Work out the finished part from the listing and answer in its coordinate system (mm). Face numbers are marked on the shaded views. A direction names the side the tool comes from. Coordinates: 2 decimals unless noted, no trailing zeros. Write each loop counter-clockwise with the first axis right and the second up, starting at its lowest first coordinate (ties: lowest second). Pieces come first, ordered by that corner, then holes. Notation, with made-up numbers: M 56.5,87.5 L 82.5,87.5 A23 cw 82.5,99.5 Z; hole C 43,39.25 d11. An arc over 180 degrees is marked long. Use CSV: the item, a comma, the result in double quotes.
from build123d import *

# Parameters (mm, degrees)
SKETCH1_W                    = 250
SKETCH1_H                    = 153
BASE_FLANGE1_DEPTH           = 2.06
EDGE_FLANGE1_STRIP_W         = 10.272
EDGE_FLANGE1_STRIP_H         = 2.06
EDGE_FLANGE1_STRIP_CUT_DEPTH = 250
EDGE_FLANGE1_DEPTH           = 250
EDGE_FLANGE2_DEPTH           = 50
CHAMFER1_SIZE                = 10
SKETCH13_R                   = 2
CUT_EXTRUDE2_DEPTH           = 8.4
SKETCH14_R                   = 2.25
CUT_EXTRUDE3_DEPTH           = 8.4
SKETCH20_W                   = 73
SKETCH20_H                   = 64
CUT_EXTRUDE9_DEPTH           = 10
FILLET1_R                    = 10
CHAMFER3_SIZE                = 15
CHAMFER4_SIZE                = 15
SKETCH21_R                   = 1.5
CUT_EXTRUDE10_DEPTH          = 10
FILLET2_R                    = 5
CUT_EXTRUDE11_DEPTH          = 10
CHAMFER5_SIZE                = 5


# Sheet-metal steps are written as plain solids
with BuildPart() as part:
    # Sketch1 → Base-Flange1 (new body)
    with BuildSketch(Plane.XY):
        with Locations((125, 76.5)):
            Rectangle(SKETCH1_W, SKETCH1_H)
    extrude(amount=-BASE_FLANGE1_DEPTH)

    # Edge-Flange1 strip (across the edge) → Edge-Flange1 strip cut (cut)
    with BuildSketch(Plane.YZ):
        with Locations((-2.06, -1.03)):
            Rectangle(EDGE_FLANGE1_STRIP_W, EDGE_FLANGE1_STRIP_H)
    extrude(amount=EDGE_FLANGE1_STRIP_CUT_DEPTH, mode=Mode.SUBTRACT)

    # Edge-Flange1 section (across the edge) → Edge-Flange1 (add)
    with BuildSketch(Plane.YZ):
        with BuildLine():
            Line((0, 1.016), (0, 15))
            Line((0, 15), (2.06, 15))
            Line((2.06, 15), (2.06, 1.016))
            ThreePointArc((2.06, 1.016), (2.35757951, 0.29757951), (3.076, 0))
            Line((3.076, 0), (3.076, -2.06))
            ThreePointArc((3.076, -2.06), (0.900939541, -1.159060459), (0, 1.016))
        make_face()
    extrude(amount=EDGE_FLANGE1_DEPTH)

    # Edge-Flange2 section (across the edge) → Edge-Flange2 (add)
    with BuildSketch(Plane(origin=(270, 87, 0), x_dir=(-1, 0, 0), z_dir=(0, 1, 0))):
        with BuildLine():
            Line((0, 1.016), (0, 15))
            Line((0, 15), (2.06, 15))
            Line((2.06, 15), (2.06, 1.016))
            ThreePointArc((2.06, 1.016), (2.35757951, 0.29757951), (3.076, 0))
            Line((3.076, 0), (20, 0))
            Line((20, 0), (20, -2.06))
            Line((20, -2.06), (3.076, -2.06))
            ThreePointArc((3.076, -2.06), (0.900939541, -1.159060459), (0, 1.016))
        make_face()
    extrude(amount=EDGE_FLANGE2_DEPTH)

    # Chamfer1
    chamfer1_edges = [part.edges().sort_by_distance(p)[0] for p in [
        (0, 1.03, 15),
        (250, 1.03, 15),
        (250, 87, -1.03),
        (250, 153, -1.03),
    ]]
    chamfer(chamfer1_edges, length=CHAMFER1_SIZE)

    # Sketch13 → Cut-Extrude2 (cut)
    with BuildSketch(Plane(origin=(0, 2.06, 0), x_dir=(1, 0, 0), z_dir=(0, 1, 0))):
        with Locations(Location((125, -8.008, 0), (0, 0, 270))):
            Circle(SKETCH13_R)
        with Locations(Location((235, -8.008, 0), (0, 0, 270))):
            Circle(SKETCH13_R)
        with Locations(Location((15, -8.008, 0), (0, 0, 270))):
            Circle(SKETCH13_R)
    extrude(amount=-CUT_EXTRUDE2_DEPTH, mode=Mode.SUBTRACT)

    # Sketch14 → Cut-Extrude3 (cut)
    with BuildSketch(Plane.ZY.offset(-267.94)):
        with Locations((8.008, 127)):
            Circle(SKETCH14_R)
        with Locations((8.008, 97)):
            Circle(SKETCH14_R)
    extrude(amount=-CUT_EXTRUDE3_DEPTH, mode=Mode.SUBTRACT)

    # Sketch20 → Cut-Extrude9 (cut)
    with BuildSketch(Plane.XY):
        with Locations((36.5, 121)):
            Rectangle(SKETCH20_W, SKETCH20_H)
    extrude(amount=-CUT_EXTRUDE9_DEPTH, mode=Mode.SUBTRACT)

    # Fillet1
    fillet1_edges = [part.edges().sort_by_distance(p)[0] for p in [
        (250, 1.03, 5),
        (240, 1.03, 15),
        (10, 1.03, 15),
        (0, 1.03, 5),
        (250, 77, -1.03),
        (260, 87, -1.03),
    ]]
    fillet(fillet1_edges, radius=FILLET1_R)

    # Chamfer3
    chamfer3_edges = [part.edges().sort_by_distance(p)[0] for p in [
        (0, 89, -1.03),
    ]]
    chamfer(chamfer3_edges, length=CHAMFER3_SIZE)

    # Chamfer4
    chamfer4_edges = [part.edges().sort_by_distance(p)[0] for p in [
        (73, 89, -1.03),
    ]]
    chamfer(chamfer4_edges, length=CHAMFER4_SIZE)

    # Sketch21 → Cut-Extrude10 (cut)
    with BuildSketch(Plane.XY):
        with Locations((27.91, 53.53)):
            Circle(SKETCH21_R)
        with Locations((207.91, 53.53)):
            Circle(SKETCH21_R)
    extrude(amount=-CUT_EXTRUDE10_DEPTH, mode=Mode.SUBTRACT)

    # Fillet2
    fillet2_edges = [part.edges().sort_by_distance(p)[0] for p in [
        (268.97, 87, 15),
        (268.97, 137, 15),
    ]]
    fillet(fillet2_edges, radius=FILLET2_R)

    # Sketch22 → Cut-Extrude11 (cut)
    with BuildSketch(Plane.XY):
        Polygon((250, 137), (250, 143), (240, 153), (73, 153), (73, 123), (225, 123), (225, 137), align=None)
    extrude(amount=-CUT_EXTRUDE11_DEPTH, mode=Mode.SUBTRACT)

    # Chamfer5
    chamfer5_edges = [part.edges().sort_by_distance(p)[0] for p in [
        (225, 137, -1.03),
        (225, 123, -1.03),
        (73, 123, -1.03),
    ]]
    chamfer(chamfer5_edges, length=CHAMFER5_SIZE)


solid = part.part
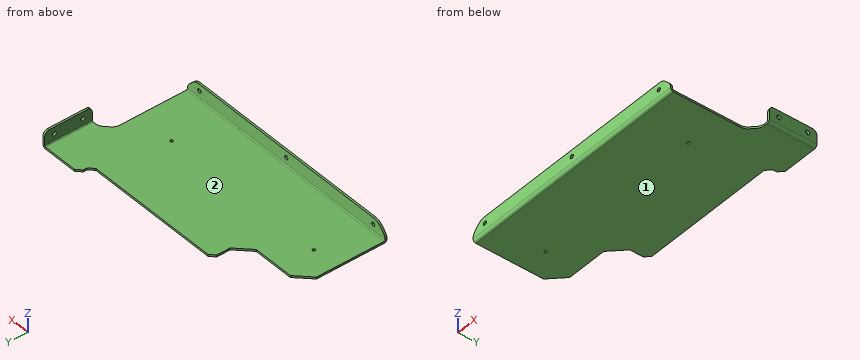
Item 1: The part is cut by section B-B (y = 108.5). Write down the section's boundary in (x, z).
Answer:
outline,"M 73,-2.06 L 266.92,-2.06 A3.08 ccw 270,1.02 L 270,15 L 267.94,15 L 267.94,1.02 A1.02 cw 266.92,0 L 73,0 Z"
Item 2: A tool of negligible diameter and unlimited length cuts with its end or side. For the marked faces 1 and 2, from which of +Z, -Z, +X, -X, +Y, -Y can it reach the whole face along a straight path? Write none if from no direction.
Answer:
face 1,"-Z, +X, -X, +Y, -Y"
face 2,"+Z, -X, +Y"
Item 3: Consider probe 1 along X at (y, z) = (71, -0.5); probe 2 along Z at (x, y) = (244.5, 128); probe 3 along Y at (x, z) = (222, 5.25). Determine where each line is inside the solid, lowest interval first.
Answer:
probe 1,"x = 0 to 250"
probe 2,"z = -2.06 to 0"
probe 3,"y = 0 to 2.06"
Item 4: Given pin 1 (1.5 mm diameter, centred on x = 126, z = 7.5, fed in from +Y); pin 2 (0.6 mm diameter, centred on y = 112.5, z = -0.5, fed in from -X); pin 3 (4 mm diameter, centred on x = 27.91, y = 53.53, fed in from +Z); pin 4 (0.6 mm diameter, centred on x = 36, z = -0.5, fed in from +Y), each flat-ended and moving along its own axis, determine where each tip first touches the part or whether it passes through.
Answer:
pin 1,"passes through"
pin 2,"stops at x = 73"
pin 3,"stops at z = 0"
pin 4,"stops at y = 89"
Item 5: The part is cut by section C-C (y = 27.5). Write down the section's boundary in (x, z), then the cut area to 3 significant figures.
Answer:
outline,"M 0,-2.06 L 250,-2.06 L 250,0 L 0,0 Z"
area,"515 mm2"
Item 6: The part is cut by section A-A (x = 160.5). Write down the section's boundary in (y, z), then the cut area to 3 significant figures.
Answer:
outline,"M 0,1.02 A3.08 ccw 3.08,-2.06 L 123,-2.06 L 123,0 L 3.08,0 A1.02 cw 2.06,1.02 L 2.06,15 L 0,15 Z"
area,"282 mm2"
